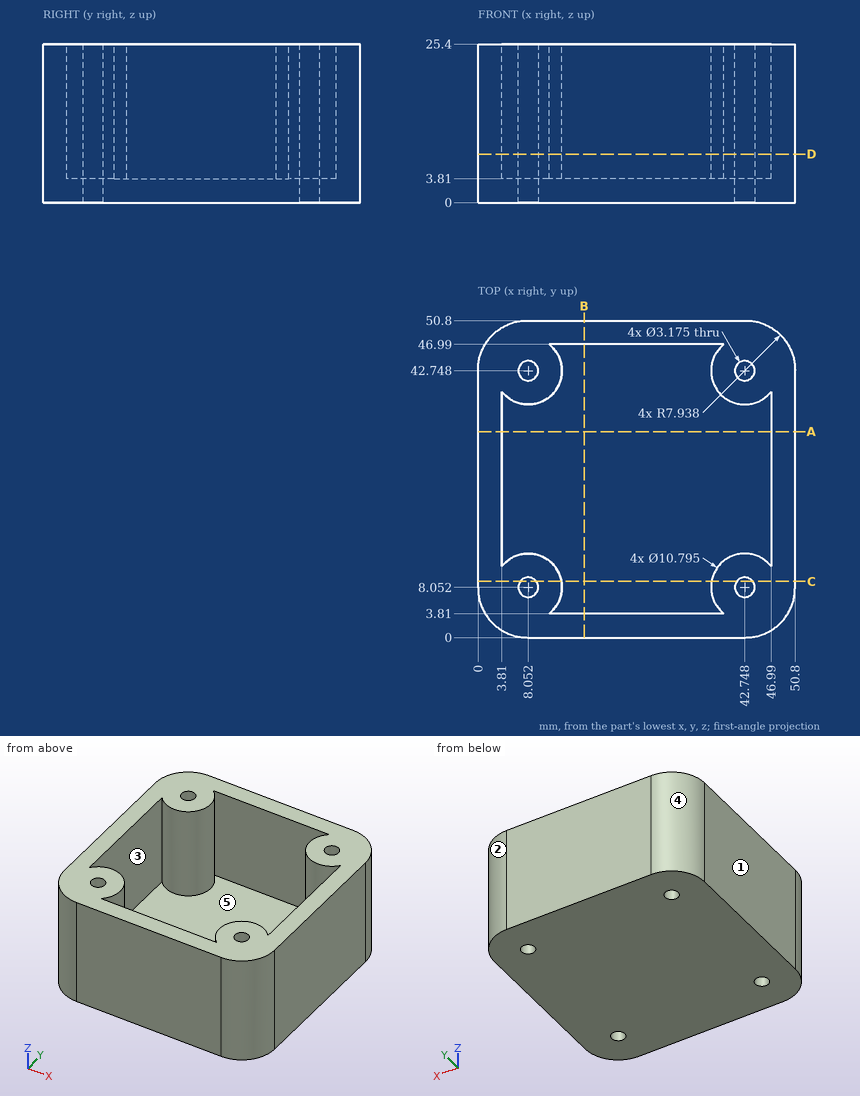
Part print with two shaded views. Sizes in mm from the minimum x, y, z corner. A direction names the side the tool comes from. Round coordinates to 2 decimals unless told otherwise and drop trailing zeros. Write each loop counter-clockwise with the first axis right and the second up, starting at its lowest first coordinate (ties: lowest second). Pieces come first, ordered by that corner, then holes. Notation, with made-up numbers: M 55.5,-24.75 L 95.5,-24.75 A22 ccw 95.5,8.25 Z; hole C 14.25,-14 d5. An arc over 180 degrees is marked long. Put each result on its own line as item: value. Start each with the question number.
1) Pull direction X, two halves, no side cores. Call the marked faces 1, 2 and 3: pulls with the +X half, pulls with the -X half, needs draft (parallel to the pull), parting line crosses it, or undercut.
2) Saw through at D-D, the plane z = 7.75. Write the cut outline in (x, y) (1 decimal).
3) Pin check, flat tips, straight feed: pin 1 Ø3 at (x, y) = (42.75, 8.05) entering from +Z; pin 2 Ø21.5 at (x, y) = (27, 22.5) entering from +Z. Stop position of each tip, or through.
4) 3-axis set-ups, long thin cutter, end or side, ignore diameter. For the marked faces 4 and 5: which of +Z, -Z, +X, -X, +Y, -Y reach the whole face in a straight line?
5) Saw through at A-A, the plane y = 33. Write the cut outline in (x, z), and give its area (3 significant figures).
6) Drill centre lines: probe 1 along Y at (x, z) = (13.5, 17.25); probe 2 along X at (y, z) = (7.5, 23.75) (1 decimal). Where is each one in solid material? Low to high. Write a range as [from, to].
7) Saw through at C-C, the plane y = 9. Write the cut outline in (x, z) (1 decimal).
Resolved:
1. face 1: pulls with the -X half
1. face 2: pulls with the +X half
1. face 3: undercut
2. outline: M 0,7.9 A7.9 ccw 7.9,0 L 42.9,0 A7.9 ccw 50.8,7.9 L 50.8,42.9 A7.9 ccw 42.9,50.8 L 7.9,50.8 A7.9 ccw 0,42.9 Z; hole M 3.8,11.4 A5.4 cw long 11.4,3.8 L 39.4,3.8 A5.4 cw long 47,11.4 L 47,39.4 A5.4 cw long 39.4,47 L 11.4,47 A5.4 cw long 3.8,39.4 Z; hole C 8.1,8.1 d3.2; hole C 8.1,42.7 d3.2; hole C 42.7,8.1 d3.2; hole C 42.7,42.7 d3.2
3. pin 1: through
3. pin 2: z = 3.81
4. face 4: +Z, -Z, -X, +Y
4. face 5: +Z
5. outline: M 0,0 L 50.8,0 L 50.8,25.4 L 46.99,25.4 L 46.99,3.81 L 3.81,3.81 L 3.81,25.4 L 0,25.4 Z
5. area: 358 mm²
6. probe 1: [0, 3.81], [46.99, 50.8]
6. probe 2: [0, 6.6], [9.5, 13.4], [37.4, 41.3], [44.2, 50.8]
7. outline: M 0,0 L 6.8,0 L 6.8,25.4 L 0,25.4 Z; M 9.3,0 L 41.5,0 L 41.5,25.4 L 37.4,25.4 L 37.4,3.8 L 13.4,3.8 L 13.4,25.4 L 9.3,25.4 Z; M 44,0 L 50.8,0 L 50.8,25.4 L 44,25.4 Z
